```python
from build123d import *

# Parameters (mm, degrees)
F0_R     = 15
F1_DEPTH = 3.5
F0_R_2   = 3
F2_DEPTH = 2


with BuildPart() as f1:
    # F0 (on Front) → F1 (new body)
    with BuildSketch(Plane.XZ):
        Circle(F0_R)
        Polygon((-4.330127, 2.5), (0, 5), (4.330127, 2.5), (4.330127, -2.5), (0, -5), (-4.330127, -2.5), align=None, mode=Mode.SUBTRACT)
    extrude(amount=F1_DEPTH)

    # F0 (on Front) → F2 (join)
    with BuildSketch(Plane.XZ):
        Circle(F0_R)
        Polygon((-4.330127, 2.5), (0, 5), (4.330127, 2.5), (4.330127, -2.5), (0, -5), (-4.330127, -2.5), align=None, mode=Mode.SUBTRACT)
        Polygon((4.330127, 2.5), (0, 5), (-4.330127, 2.5), (-4.330127, -2.5), (0, -5), (4.330127, -2.5), align=None)
        Circle(F0_R_2, mode=Mode.SUBTRACT)
    extrude(amount=-F2_DEPTH)


solid = f1.part
```
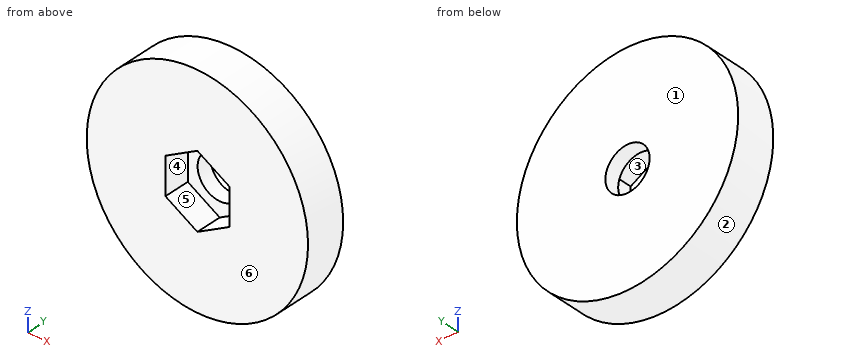
The model under review builds one solid part; all positions refer to its coordinate system, in mm. Face numbers are marked on the shaded views. A direction names the side the tool comes from. Coordinates: 2 decimals unless noted, no trailing zeros. Write each loop counter-clockwise with the first axis right and the second up, starting at its lowest first coordinate (ties: lowest second). Pieces come first, ordered by that corner, then holes.
1) The part is to be moulded in two halves that separate along Z. For the marked faces 1, 2, 3 and 4, say which applies: pulls with the +Z half, pulls with the -Z half, needs draft (parallel to the pull), parting line crosses it, or undercut.
2) We need section C-C on x = 1.75. State the section outline as (y, z) points.
3) To check wall thickness, follow probe 1 along Z at (x, y) = (0, 1.3); probe 2 along Z at (x, y) = (-3.5, -3.05); probe 3 along X at (y, z) = (1.35, -5.75). State the ranges of each line that lie inside material, in increasing order.
4) We need section A-A on z = 0. State the section outline as (x, y) points.
5) Clearance check with flat-ended pins moving along their axes: pin 1 Ø1 at (y, z) = (-2, 1) entering from +X; pin 2 Ø1.5 at (y, z) = (1, 8) entering from -X; pin 3 Ø2.5 at (x, z) = (0, 2) entering from -Y. State where each tip first meets the part, or that it passes through.
6) We need section B-B on y = -1.3. State the section outline as (x, z) points.
7) We need section D-D on x = -3.5. State the section outline as (y, z) points.
8) Machinability: for the marked faces 5 and 6, which of the approach directions +Z, -Z, +X, -X, +Y, -Y give a long, thin tool a straight path to every point of the face, cutting with its end or side? Answer none if there is none.
Answer list:
1. face 1: needs draft
1. face 2: parting line crosses it
1. face 3: undercut
1. face 4: undercut
2. outline: (-3.5, -14.9) - (2, -14.9) - (2, -2.44) - (0, -2.44) - (0, -3.99) - (-3.5, -3.99) - close; (-3.5, 3.99) - (0, 3.99) - (0, 2.44) - (2, 2.44) - (2, 14.9) - (-3.5, 14.9) - close
3. probe 1: z = -15 to -3, 3 to 15
3. probe 2: z = -14.59 to -2.98, 2.98 to 14.59
3. probe 3: x = -13.85 to 13.85
4. outline: (-15, -3.5) - (-4.33, -3.5) - (-4.33, 0) - (-3, 0) - (-3, 2) - (-15, 2) - close; (3, 0) - (4.33, 0) - (4.33, -3.5) - (15, -3.5) - (15, 2) - (3, 2) - close
5. pin 1: stops at x = 14.99
5. pin 2: stops at x = -13.13
5. pin 3: stops at y = 0
6. outline: circle Ø30 at (0, 0); hole (-4.33, -2.5) - (0, -5) - (4.33, -2.5) - (4.33, 2.5) - (0, 5) - (-4.33, 2.5) - close
7. outline: (-3.5, -14.59) - (2, -14.59) - (2, 14.59) - (-3.5, 14.59) - (-3.5, 2.98) - (0, 2.98) - (0, -2.98) - (-3.5, -2.98) - close
8. face 5: -Y
8. face 6: +Z, -Z, +X, -X, -Y
